Verification items for the finished model (mm, model axes). Coordinates: 2 decimals unless noted, no trailing zeros. Order: outer loops, then holes, each group sorted by start corner. A loop starts at its lowest first (then second) coordinate and runs counter-clockwise, first axis right, second up. Notation, with made-up numbers: (47, 38) -> (89, 38) arc R17 cw to (89, 66) -> close; hole circle Ø4 at (-12, 7.5). An arc over 180 degrees is marked (long way). Write item = value, one per line. Start each with the question number.
from build123d import *

# Parameters (mm, degrees)
F0_R     = 11.05
F0_R_2   = 13.55
F1_DEPTH = 7


with BuildPart() as f1:
    # F0 (on Top) → F1 (new body)
    with BuildSketch(Plane.XY):
        with BuildLine():
            ThreePointArc((-10.021513, -13.654951), (-14.364957, -3.713029), (-24.610712, -0.14486))
            ThreePointArc((-24.610712, -0.14486), (-35.500503, -20.081591), (-12.860881, -21.954642))
            ThreePointArc((-12.860881, -21.954642), (-10.750991, -18.04092), (-10.021513, -13.654951))
        make_face()
        with Locations((-23.571513, -13.654951)):
            Circle(F0_R, mode=Mode.SUBTRACT)
        with BuildLine():
            ThreePointArc((13.423732, 25.728168), (13.518396, 26.648767), (13.55, 27.573681))
            ThreePointArc((13.55, 27.573681), (-0.81156, 41.099355), (-13.452785, 25.953474))
            add(Edge.make_bspline(
                [(-13.036801, 23.87986), (-13.14978, 24.554538), (-13.288064, 25.245532), (-13.452785, 25.953474)],
                knots=[26.868894, 26.868894, 26.868894, 26.868894, 28.383488, 28.383488, 28.383488, 28.383488], degree=3))
            ThreePointArc((-13.036801, 23.87986), (0.944187, 14.056617), (13.423732, 25.728168))
        make_face()
        with Locations((0, 27.573681)):
            Circle(F0_R, mode=Mode.SUBTRACT)
        with BuildLine():
            ThreePointArc((37.469286, -13.454165), (34.0534, -4.459598), (25.527997, 0))
            ThreePointArc((25.527997, 0), (12.257933, -6.553778), (12.900423, -21.340049))
            ThreePointArc((12.900423, -21.340049), (28.060355, -26.355872), (37.469286, -13.454165))
        make_face()
        with Locations((23.919286, -13.454165)):
            Circle(F0_R, mode=Mode.SUBTRACT)
        with BuildLine():
            add(Edge.make_bspline(
                [(13.423732, 25.728168), (11.58878, 7.021586), (15.626226, 7.021586), (25.527997, 0)],
                knots=[0, 0, 0, 0, 28.433288, 28.433288, 28.433288, 28.433288], degree=3))
            ThreePointArc((13.423732, 25.728168), (0.944187, 14.056617), (-13.036801, 23.87986))
            add(Edge.make_bspline(
                [(-24.610712, -0.14486), (-16.992516, 5.077212), (-11.032568, 11.911073), (-13.036801, 23.87986)],
                knots=[0, 0, 0, 0, 26.868894, 26.868894, 26.868894, 26.868894], degree=3))
            ThreePointArc((-24.610712, -0.14486), (-14.364957, -3.713029), (-10.021513, -13.654951))
            ThreePointArc((-10.021513, -13.654951), (-10.750991, -18.04092), (-12.860881, -21.954642))
            add(Edge.make_bspline(
                [(-12.860881, -21.954642), (-2.93959, -15.780944), (3.867878, -15.780944), (12.900423, -21.340049)],
                knots=[0, 0, 0, 0, 25.768635, 25.768635, 25.768635, 25.768635], degree=3))
            ThreePointArc((12.900423, -21.340049), (12.257933, -6.553778), (25.527997, 0))
        make_face()
        Circle(F0_R_2, mode=Mode.SUBTRACT)
        Circle(F0_R_2)
        Circle(F0_R, mode=Mode.SUBTRACT)
    extrude(amount=F1_DEPTH)


solid = f1.part
Item 1: Section check A-A (y = -1). Record the boundary of the cut face in (x, z).
Item 2: Gauge pin test, flat ends, axial feed: P1, Ø3, axis at y = 31, z = 6, coming from the +X side; P2, Ø1, axis at x = -8, y = 6, coming from the -Z side; P3, Ø3, axis at x = 10, z = 3, coming from the -Y side; P4, Ø4, axis at x = -25, z = 3.5, coming from the +Y side. Record the tip position at first contact, or that the pin passes through.
Item 3: Mould release check, pull along X, two halves, no side actions. Record for faces 1 (the cylindrical face through (-0.503, 41.114, 3.451)), 2 (the cylindrical face through (-2.395, -10.787, 3.451)), 3 (the flat face through (-6, 10, 0)), 4 (the cylindrical face through (13.518, 26.636, 3.451)): pulls with the +X half, pulls with the -X half, needs draft (parallel to the pull), parting line crosses it, or undercut.
Item 4: Section check B-B (x = 0). State how many separate pieces and enclosed holes the cut face has, then the cut area to 3 significant figures.
Item 5: Thickness scan on line 1 (Y direction, x = 0, z = 3.25); line 2 (Y direction, x = 7.5, z = 6.75); line 3 (X direction, y = -5, z = 4). Record the ranges inside material, lowest first.
Filled sheet:
q1.outline = (-28.41, 0) -> (-11, 0) -> (-11, 7) -> (-28.41, 7) -> close; (11, 0) -> (29.26, 0) -> (29.26, 7) -> (11, 7) -> close
q2.P1 = 13.41
q2.P2 = through
q2.P3 = -20.51
q2.P4 = 1
q3.face_1 = parting line crosses it
q3.face_2 = undercut
q3.face_3 = needs draft
q3.face_4 = pulls with the +X half
q4.separate_pieces = 3
q4.enclosed_holes = 0
q4.area = 99.3 mm^2
q5.line_1 = -17.26 to -11.05, 11.05 to 16.52, 38.62 to 41.12
q5.line_2 = -18.6 to -8.11, 8.11 to 19.46, 35.69 to 38.86
q5.line_3 = -34 to -30.44, -16.7 to -9.85, 9.85 to 16.8, 31.03 to 34.51
